Geometry check sheet. Reference: the model listing, model coordinates, mm. Give positions to 0.01 mm unless a question says otherwise; leave off trailing zeros. Order: outer loops, then holes, each group sorted by start corner. A loop starts at its lowest first (then second) coordinate and runs counter-clockwise, first axis right, second up. Notation, with made-up numbers: M -24,56 L 3,56 A11 cw 3,65 Z; hole C 83,80.5 d4. An arc over 180 degrees is marked long. Answer as CSV lines item,"result". Start each with the question number.
```python
from build123d import *

# Parameters (mm, degrees)
SKETCH1_R           = 1.3
BOSS_EXTRUDE1_DEPTH = 2.5


with BuildPart() as part:
    # Sketch1 → Boss-Extrude1 (new body)
    with BuildSketch(Plane(origin=(0, 0, 0), x_dir=(1, 0, 0), z_dir=(0, 1, 0))):
        with BuildLine():
            ThreePointArc((16, 0), (-12.25671109, -10.284601755), (2.778370843, 15.756924048))
            Line((2.778370843, 15.756924048), (4.775324886, 27.082213208))
            ThreePointArc((4.775324886, 27.082213208), (-21.066222186, -17.676659266), (27.5, 0))
            ThreePointArc((27.5, 0), (27.395354198, 2.396782926), (27.082213208, 4.775324886))
            Line((27.082213208, 4.775324886), (15.756924048, 2.778370843))
            ThreePointArc((15.756924048, 2.778370843), (15.939115169, 1.394491884), (16, 0))
        make_face()
        with Locations(Location((0, -24.3, 0), (0, 0, 270))):
            Circle(SKETCH1_R, mode=Mode.SUBTRACT)
        with Locations(Location((0, -18.5, 0), (0, 0, 270))):
            Circle(SKETCH1_R, mode=Mode.SUBTRACT)
        with Locations(Location((-24.3, 0, 0), (0, 0, 270))):
            Circle(SKETCH1_R, mode=Mode.SUBTRACT)
        with Locations(Location((-18.5, 0, 0), (0, 0, 270))):
            Circle(SKETCH1_R, mode=Mode.SUBTRACT)
        with Locations(Location((0, 18.5, 0), (0, 0, 270))):
            Circle(SKETCH1_R, mode=Mode.SUBTRACT)
        with Locations(Location((18.5, 0, 0), (0, 0, 270))):
            Circle(SKETCH1_R, mode=Mode.SUBTRACT)
        with Locations(Location((24.3, 0, 0), (0, 0, 270))):
            Circle(SKETCH1_R, mode=Mode.SUBTRACT)
        with Locations(Location((0, 24.3, 0), (0, 0, 270))):
            Circle(SKETCH1_R, mode=Mode.SUBTRACT)
    extrude(amount=BOSS_EXTRUDE1_DEPTH)


solid = part.part
```
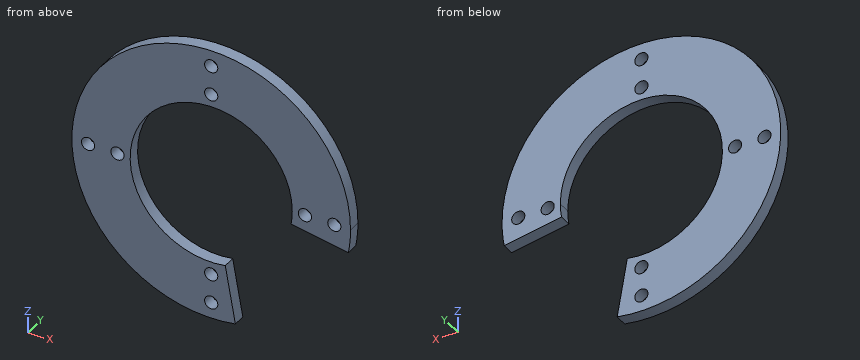
Item 1: Section check C-C on y = 1.1. Give the number of separate pieces and of enclosed holes in the cut face, then the cut area to 3 significant figures.
Item 2: Section check D-D on z = -13. Record the boundary of the cut face in (x, y), then the cut area to 3 significant figures.
Item 3: Section check B-B on z = 8. Record the boundary of the cut face in (x, y), then the cut area to 3 significant figures.
Item 4: Depth check by flat-ended pin: pin 1 Ø1 at (y, z) = (1.5, -16.5) entering from -X. Enter the tip coordinate at first touch or a pass-through.
Item 5: Section check A-A on x = 18.5. Record the boundary of the cut face in (y, z), then the cut area to 3 significant figures.
Item 6: Scan lines: line 1 along Z through (x, y) = (1, 1.85); line 2 along X through (y, z) = (1.8, 24.3). Record each from-to range of solid material in increasing order.
Numbers:
1,separate pieces,"1"
1,enclosed holes,"8"
1,area,"1,220 mm2"
2,outline,"M -24.23,0 L -9.33,0 L -9.33,2.5 L -24.23,2.5 Z"
2,area,"37.3 mm2"
3,outline,"M -26.31,0 L -13.86,0 L -13.86,2.5 L -26.31,2.5 Z; M 13.86,0 L 26.31,0 L 26.31,2.5 L 13.86,2.5 Z"
3,area,"62.3 mm2"
4,pin 1,"x = -22.37"
5,outline,"M 0,-3.26 L 2.5,-3.26 L 2.5,-1.3 L 0,-1.3 Z; M 0,1.3 L 2.5,1.3 L 2.5,20.35 L 0,20.35 Z"
5,area,"52.5 mm2"
6,line 1,"-27.48 to -25.13, -23.47 to -19.33, -17.67 to -15.97, 15.97 to 17.67, 19.33 to 23.47, 25.13 to 27.48"
6,line 2,"-12.87 to -1.3, 1.3 to 12.87"
